Design review of the part built by this model. Coordinates are the model's own, in mm. A direction names the side the tool comes from. Give positions to 0.01 mm unless a question says otherwise; leave off trailing zeros. Loops run counter-clockwise (first coordinate to the right, second up) from the corner with the lowest first, then second, coordinate; pieces in that order, holes last. Notation, with made-up numbers: (25, 22.25) -> (62, 22.25) arc R17 cw to (62, 36.25) -> close; hole circle Ø10 at (32, 83.25). An arc over 180 degrees is marked (long way). Use a Markdown table: item, result. Add a question column.
1. Add section B-B (x = 23). State the section outline as (y, z) points (3 decimals).
2. For faces 1 (the flat face through (-28, 4, 9.525)), 2 (the flat face through (0, -304.8, 71)), 3 (the flat face through (27, 4, 9.525)), list the 3-axis set-ups (+Z, -Z, +X, -X, +Y, -Y) from which the entire face can be reached by the end or side of a thin tool; tool diameter is ignored.
3. To check wall thickness, follow line 1 (Z direction, x = 27.5, y = -203) (3 decimals); line 2 (X direction, y = -277.5, z = 60). State the ranges of each line that lie inside material, in increasing order.
4. Add section A-A (y = 105). State the section outline as (x, z) points (1 decimal), and give its area (3 significant figures).
5. For pin 1 Ø8 at (x, y) = (23.5, -157.5) entering from -Z; pin 2 Ø12 at (y, z) = (198, 181) entering from +X; pin 3 Ø23.5 at (x, y) = (-27, 33) entering from +Z (3 decimals); pin 4 Ø1.5 at (y, z) = (-139, 140) entering from -X, all flat-tipped, find the tip position at first contact; note any pin that passes through.
6. Add section C-C (z = 104.5). State the section outline as (x, y) points.
```python
from build123d import *

# Parameters (mm, degrees)
BOSS_EXTRUDE1_DEPTH = 304.8
FILLET1_R           = 152.4


with BuildPart() as part:
    # Sketch1 → Boss-Extrude1 (new body, symmetric)
    with BuildSketch(Plane(origin=(0, 0, 0), x_dir=(-1, 0, 0), z_dir=(0, 1, 0))):
        Polygon((-50.8, 0), (50.8, 0), (50.8, 9.525), (3.96875, 9.525), (3.96875, 201.6125), (-3.96875, 201.6125), (-3.96875, 9.525), (-50.8, 9.525), align=None)
    extrude(amount=BOSS_EXTRUDE1_DEPTH, both=True)

    # Fillet1
    fillet1_edges = [part.edges().sort_by_distance(p)[0] for p in [
        (0, 304.8, 201.6125),
    ]]
    fillet(fillet1_edges, radius=FILLET1_R)


solid = part.part
```
Taken from the geometry:
| question | item | result |
|---|---|---|
| 1 | outline | (-304.8, 0) -> (304.8, 0) -> (304.8, 9.525) -> (-304.8, 9.525) -> close |
| 2 | face 1 | +Z, -X, +Y, -Y |
| 2 | face 2 | +Z, -Z, +X, -X, -Y |
| 2 | face 3 | +Z, +X, +Y, -Y |
| 3 | line 1 | z = 0 to 9.525 |
| 3 | line 2 | x = -3.97 to 3.97 |
| 4 | outline | (-50.8, 0) -> (50.8, 0) -> (50.8, 9.5) -> (4, 9.5) -> (4, 201.6) -> (-4, 201.6) -> (-4, 9.5) -> (-50.8, 9.5) -> close |
| 4 | area | 2,490 mm^2 |
| 5 | pin 1 | stops at z = 0 |
| 5 | pin 2 | stops at x = 3.97 |
| 5 | pin 3 | stops at z = 9.525 |
| 5 | pin 4 | stops at x = -3.97 |
| 6 | outline | (-3.97, -304.8) -> (3.97, -304.8) -> (3.97, 294.42) -> (-3.97, 294.42) -> close |
